Geometry: see drawing. Coordinates: mm, zero at the bounding-box minimum. A direction names the side the tool comes from. Give positions to 0.01 mm unless a question says otherwise; leave off trailing zeros. Loops run counter-clockwise (first coordinate to the right, second up) from the corner with the lowest first, then second, coordinate; pieces in that order, holes last. Notation, with made-up numbers: M -14.5,-1 L -2.5,-1 A21 cw -2.5,27 Z; hole C -5.5,49.25 d9. An arc over 180 degrees is marked long. Put each result on its own line as item: value.
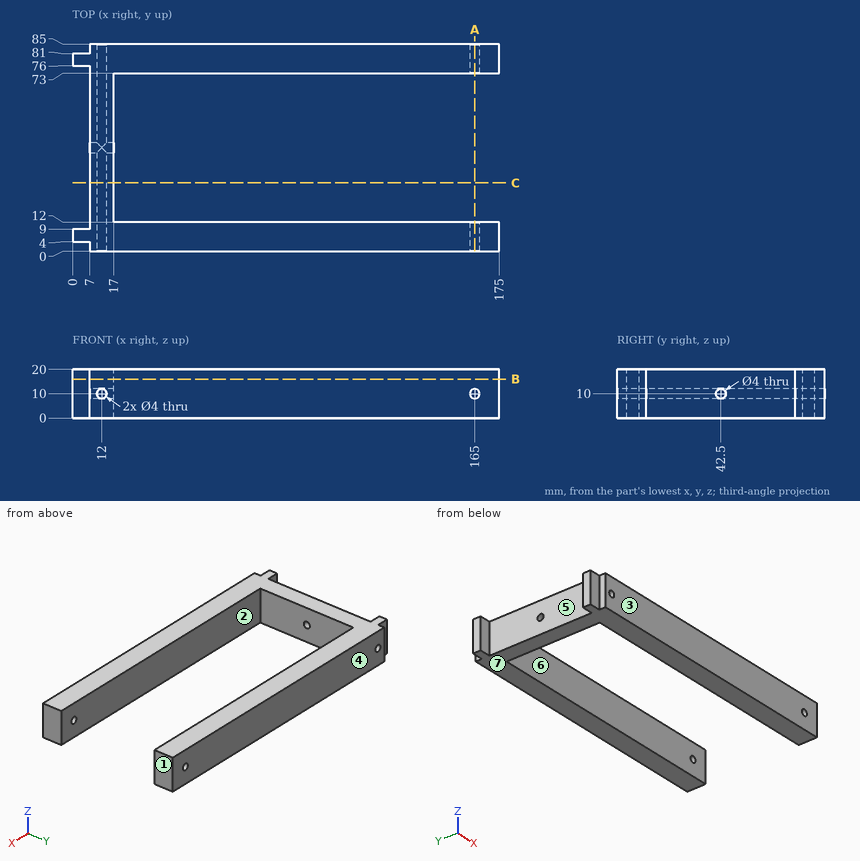
1. Draft query along Y for the marked faces 1, 2, 3 and 4. Return one class per face: pulls with the +Y half, pulls with the -Y half, needs draft (parallel to the pull), parting line crosses it, or undercut.
Found:
face 1: needs draft
face 2: undercut
face 3: pulls with the -Y half
face 4: pulls with the +Y half
2. Contact query for flat-ended pins moving along their axis: P1, Ø1, axis at y = 12.5, z = 7, coming from the -X side; P2, Ø8, axis at y = 65, z = 10, coming from the +X side; P3, Ø2, axis at x = 4.5, z = 9.5, coming from the +Y side. Output: stop coordinate, or through.
Found:
P1: x = 7
P2: x = 17
P3: y = 81
3. Access query for the marked faces 5, 6 and 7. Directions: +Z, -Z, +X, -X, +Y, -Y. A direction counts if a zero-diameter tool reaches every point of the face in a straight line with its end or side. Return the directions, or none.
Found:
face 5: +Z, -Z, -X
face 6: +Z, -Z, +X
face 7: -Z, +X, -X, +Y, -Y
4. Section query C-C (y = 28). Output: boundary loops of the cut face in (x, z), plus the area to 3 significant figures.
Found:
outline: M 7,0 L 17,0 L 17,20 L 7,20 Z; hole C 12,10 d4
area: 187 mm^2
5. Section query B-B (z = 16). Output: boundary loops of the cut face in (x, y).
Found:
outline: M 0,4 L 7,4 L 7,0 L 175,0 L 175,12 L 17,12 L 17,73 L 175,73 L 175,85 L 7,85 L 7,81 L 0,81 L 0,76 L 7,76 L 7,9 L 0,9 Z
6. Material intervals for line 1 (Y direction, x = 81, z = 18.5); line 2 (Y direction, x = 8.9, z = 10); line 3 (X direction, y = 32, z = 10), sorted ascending. Write a range as from..to.
Found:
line 1: 0..12, 73..85
line 2: 0..40.5, 44.5..85
line 3: 7..10, 14..17
7. Section query A-A (x = 165). Output: boundary loops of the cut face in (y, z).
Found:
outline: M 0,0 L 12,0 L 12,8 L 0,8 Z; M 0,12 L 12,12 L 12,20 L 0,20 Z; M 73,0 L 85,0 L 85,8 L 73,8 Z; M 73,12 L 85,12 L 85,20 L 73,20 Z
